Source: CAD feature listing. Evaluate the final solid. Frame: model axes, mm. A direction names the side the tool comes from. Round coordinates to 2 decimals unless told otherwise and drop trailing zeros. Loops run counter-clockwise (first coordinate to the right, second up) from the corner with the lowest first, then second, coordinate; pieces in that order, holes last. Notation, with made-up numbers: M -0.5,68 L 11.5,68 A26 ccw 11.5,105 Z; hole C 83.25,-39 d5. An arc over 180 degrees is marked long. Write each question's results on one line, items separated by ' | '. Start each with the question number.
1. Section B-B on z = 8. Give the number of separate pieces and of enclosed holes in the cut face, and give its area (3 significant figures).
2. Ray query, line 1 (Y direction, x = 33.5, z = 11.5); line 2 (X direction, y = 17.5, z = 2.25); line 3 (X direction, y = 18.5, z = 5.25). Return the intervals inside material, ascending.
3. Draft query along X for faces 1 (the flat face through (33, 19, 12.7)), 2 (the cylindrical face through (113.13, 27.85, 14.73)). Return one class per face: released by +X, released by -X, zero draft, split by the parting line, or undercut.
4. Section A-A on x = 78. Output: boundary loops of the cut face in (y, z), and give its area (3 significant figures).
5. Set-up query: faces 3 (the cylindrical face through (136.763, 7.24, 5.151)), 4 (the flat face through (120, 6, 12.7)), 5 (the cylindrical face through (80.8, 20.1, 11.4)), 6 (the flat face through (62, 0, 5)), 7 (the flat face through (77, 25.146, 5)). Return all of +Z, -Z, +X, -X, +Y, -Y with unobstructed straight access to the full face (end or side cutting, diameter ignored); none if empty.
6. Section C-C on x = 119. Output: boundary loops of the cut face in (y, z).
7. Contact query for flat-ended pins moving along their axis: pin 1 Ø3.5 at (x, y) = (31, 9.5) entering from +Z; pin 2 Ø5 at (x, z) = (106, 3.5) entering from +Y; pin 3 Ø8 at (x, z) = (65.5, 5) entering from -Y; pin 4 Ø2 at (x, z) = (19, 8) entering from -Y. Output: stop coordinate, or through.
from build123d import *

# Parameters (mm, degrees)
SKETCH1_W           = 139.7
SKETCH1_H           = 25.146
BOSS_EXTRUDE1_DEPTH = 10.16
SKETCH3_W           = 2.794
SKETCH3_H           = 32.004
BOSS_EXTRUDE2_DEPTH = 15.494
FILLET1_R           = 2.54
SKETCH4_R           = 4.064
BOSS_EXTRUDE3_DEPTH = 2.54
SKETCH5_R           = 2.54
SKETCH5_R_2         = 3.1496
CUT_EXTRUDE1_DEPTH  = 10.16


with BuildPart() as part:
    # Sketch1 → Boss-Extrude1 (new body)
    with BuildSketch(Plane.XY):
        with Locations((69.85, 12.573)):
            Rectangle(SKETCH1_W, SKETCH1_H)
    extrude(amount=BOSS_EXTRUDE1_DEPTH)

    # Sketch3 → Boss-Extrude2 (add)
    with BuildSketch(Plane.XY):
        with Locations((98.6282, 12.573)):
            Rectangle(SKETCH3_W, SKETCH3_H)
        with Locations((127.5842, 12.573)):
            Rectangle(SKETCH3_W, SKETCH3_H)
        with Locations((113.1062, 12.573)):
            Rectangle(SKETCH3_W, SKETCH3_H)
        with Locations((84.1502, 12.573)):
            Rectangle(SKETCH3_W, SKETCH3_H)
        with Locations((69.6722, 12.573)):
            Rectangle(SKETCH3_W, SKETCH3_H)
        with Locations((55.1942, 12.573)):
            Rectangle(SKETCH3_W, SKETCH3_H)
        with Locations((40.7162, 12.573)):
            Rectangle(SKETCH3_W, SKETCH3_H)
        with Locations((26.2382, 12.573)):
            Rectangle(SKETCH3_W, SKETCH3_H)
        with Locations((11.7602, 12.573)):
            Rectangle(SKETCH3_W, SKETCH3_H)
    extrude(amount=BOSS_EXTRUDE2_DEPTH)

    # Fillet1
    fillet1_edges = [part.edges().sort_by_distance(p)[0] for p in [
        (69.6722, -3.429, 15.494),
        (69.6722, 28.575, 15.494),
        (55.1942, -3.429, 15.494),
        (55.1942, 28.575, 15.494),
        (40.7162, -3.429, 15.494),
        (40.7162, 28.575, 15.494),
        (26.2382, -3.429, 15.494),
        (26.2382, 28.575, 15.494),
        (11.7602, -3.429, 15.494),
        (11.7602, 28.575, 15.494),
        (127.5842, -3.429, 15.494),
        (127.5842, 28.575, 15.494),
        (113.1062, -3.429, 15.494),
        (113.1062, 28.575, 15.494),
        (98.6282, -3.429, 15.494),
        (98.6282, 28.575, 15.494),
        (84.1502, -3.429, 15.494),
        (84.1502, 28.575, 15.494),
    ]]
    fillet(fillet1_edges, radius=FILLET1_R)

    # Sketch4 → Boss-Extrude3 (add)
    with BuildSketch(Plane.XY.offset(10.16)):
        with Locations((18.9992, 18.923)):
            Circle(SKETCH4_R)
        with Locations((18.9992, 6.223)):
            Circle(SKETCH4_R)
        with Locations((47.9552, 18.923)):
            Circle(SKETCH4_R)
        with Locations((47.9552, 6.223)):
            Circle(SKETCH4_R)
        with Locations((33.4772, 18.923)):
            Circle(SKETCH4_R)
        with Locations((33.4772, 6.223)):
            Circle(SKETCH4_R)
        with Locations((62.4332, 18.923)):
            Circle(SKETCH4_R)
        with Locations((62.4332, 6.223)):
            Circle(SKETCH4_R)
        with Locations((76.9112, 18.923)):
            Circle(SKETCH4_R)
        with Locations((76.9112, 6.223)):
            Circle(SKETCH4_R)
        with Locations((91.3892, 18.923)):
            Circle(SKETCH4_R)
        with Locations((91.3892, 6.223)):
            Circle(SKETCH4_R)
        with Locations((105.8672, 18.923)):
            Circle(SKETCH4_R)
        with Locations((105.8672, 6.223)):
            Circle(SKETCH4_R)
        with Locations((120.3452, 18.923)):
            Circle(SKETCH4_R)
        with Locations((120.3452, 6.223)):
            Circle(SKETCH4_R)
    extrude(amount=BOSS_EXTRUDE3_DEPTH)

    # Sketch5 → Cut-Extrude1 (cut)
    with BuildSketch(Plane.XY.offset(10.16)):
        with Locations((5.1816, 18.669)):
            Circle(SKETCH5_R)
        with Locations((134.3406, 18.669)):
            Circle(SKETCH5_R)
        with Locations((134.3406, 12.573)):
            Circle(SKETCH5_R_2)
        with Locations((5.1816, 6.477)):
            Circle(SKETCH5_R)
        with Locations((134.3406, 6.477)):
            Circle(SKETCH5_R)
        with Locations((5.1816, 12.573)):
            Circle(SKETCH5_R_2)
    extrude(amount=-CUT_EXTRUDE1_DEPTH, mode=Mode.SUBTRACT)


solid = part.part
Taken from the geometry:
1) separate pieces: 1 | enclosed holes: 6 | area: 3,540 mm^2
2) line 1: 2.16 to 10.29, 14.86 to 22.99 | line 2: 0 to 2.93, 7.44 to 132.09, 136.6 to 139.7 | line 3: 0 to 2.65, 7.72 to 131.81, 136.87 to 139.7
3) face 1: undercut | face 2: zero draft
4) outline: M 0,0 L 25.15,0 L 25.15,10.16 L 22.84,10.16 L 22.84,12.7 L 15.01,12.7 L 15.01,10.16 L 10.14,10.16 L 10.14,12.7 L 2.31,12.7 L 2.31,10.16 L 0,10.16 Z | area: 295 mm^2
5) face 3: +Z, -Z | face 4: +Z, +Y, -Y | face 5: +Z | face 6: +Z, -Z, -Y | face 7: +Z, -Z, +Y
6) outline: M 0,0 L 25.15,0 L 25.15,10.16 L 22.76,10.16 L 22.76,12.7 L 15.09,12.7 L 15.09,10.16 L 10.06,10.16 L 10.06,12.7 L 2.39,12.7 L 2.39,10.16 L 0,10.16 Z
7) pin 1: z = 12.7 | pin 2: y = 25.15 | pin 3: y = -3.43 | pin 4: y = 0
